from build123d import *

# Parameters (mm, degrees)
BOSS_EXTRUDE3_DEPTH      = 20
BOSS_EXTRUDE3_DEPTH_BACK = 90
SKETCH5_R                = 5


with BuildPart() as part:
    # Sketch4 → Revolve1 (revolve)
    with BuildSketch(Plane.XY, mode=Mode.PRIVATE) as revolve1_sk:
        with BuildLine():
            Line((0, 0), (75, 0))
            Line((75, 0), (75, 35))
            Line((75, 35), (72.5, 35))
            ThreePointArc((72.5, 35), (62.5, 25), (52.5, 35))
            Line((52.5, 35), (50, 35))
            Line((50, 35), (50, 25))
            Line((50, 25), (0, 25))
            Line((0, 25), (0, 0))
        make_face()
    revolve(revolve1_sk.sketch.rotate(Axis((0, 0, 0), (1, 0, 0)), 90), axis=Axis((0, 0, 0), (1, 0, 0)))

    # Sketch5 → Boss-Extrude3 (add, two sides: drawn at the far end of the back side and taken through both)
    with BuildSketch(Plane(origin=(75, 0, 0), x_dir=(0, 0, -1), z_dir=(1, 0, 0)).offset(-BOSS_EXTRUDE3_DEPTH_BACK)):
        Circle(SKETCH5_R)
    extrude(amount=BOSS_EXTRUDE3_DEPTH + BOSS_EXTRUDE3_DEPTH_BACK)


solid = part.part
The listing builds one solid part. Answer for the finished solid, in the listing's coordinates (mm). A direction names the side the tool comes from. Give positions to 0.01 mm unless a question says otherwise; leave off trailing zeros. Write each loop counter-clockwise with the first axis right and the second up, starting at its lowest first coordinate (ties: lowest second). Pieces come first, ordered by that corner, then holes. Notation, with made-up numbers: (19.5, 24.5) - (62.5, 24.5) arc R24 ccw to (62.5, 53.5) - close; hole circle Ø4 at (85, -36.5). An arc over 180 degrees is marked (long way). One line per question, with ' | ' between items. Start each with the question number.
1. Section C-C, the plane x = 81.5 is taken. Determine the outline of the cut face in (y, z).
2. For faces 1 (the face through (84.86, -4.88, 1.08)), 2 (the face through (51.232, 34.168, -7.587)), 3 (the face through (24.65, -7.509, 23.846)), determine the directions among +Z, -Z, +X, -X, +Y, -Y from which every point of the face is accessible in a straight line to the end or side of a thin tool.
3. Straight lines are drawn through the part: line 1 (X direction, y = 32, z = -12.5); line 2 (X direction, y = 30.5, z = 2); line 3 (X direction, y = 11, z = -9). For each, find the intervals that lie inside material, in ascending order.
4. Section A-A, the plane y = 0 is taken. Determine the outline of the cut face in (x, z), then the cut area to 3 significant figures.
5. Given P1, Ø12, axis at x = 53.5, z = 6.5, coming from the -Y side; P2, Ø25, axis at y = 7.5, z = 5, coming from the -X side; P3, Ø3, axis at y = 24.5, z = -15, coming from the +X side; P4, Ø8, axis at x = 79.5, z = -7.5, coming from the -Y side, each flat-ended and moving along its own axis, determine where each tip first touches the part or whether it passes through.
6. Section D-D, the plane x = 7 is taken. Determine the outline of the cut face in (y, z), then the cut area to 3 significant figures.
Result:
1) outline: circle Ø10 at (0, 0)
2) face 1: +X | face 2: +X, -X | face 3: -X
3) line 1: x = 50 to 52.52, 72.48 to 75 | line 2: x = 50 to 53.54, 71.46 to 75 | line 3: x = 0 to 75
4) outline: (-15, -5) - (0, -5) - (0, -25) - (50, -25) - (50, -35) - (52.5, -35) arc R10 cw to (72.5, -35) - (75, -35) - (75, -5) - (95, -5) - (95, 5) - (75, 5) - (75, 35) - (72.5, 35) arc R10 cw to (52.5, 35) - (50, 35) - (50, 25) - (0, 25) - (0, 5) - (-15, 5) - close | area: 4,290 mm2
5) P1: stops at y = -35 | P2: stops at x = -15 | P3: stops at x = 75 | P4: stops at y = -3.57
6) outline: circle Ø50 at (0, 0) | area: 1,960 mm2
